from build123d import *

# Parameters (mm, degrees)
SKETCH_1_R           = 305
EXTRUDE_1_DEPTH      = 41.2
SKETCH_4_W           = 140
SKETCH_4_H           = 140
EXTRUDE_2_DEPTH      = 10
SHELL_1_T            = -5
CUT_EXTRUDE_3_DEPTH  = 434.298326791
SKETCH_5_R           = 8
SKETCH_5_R_2         = 4
CUT_EXTRUDE_6_DEPTH  = 435.363258115
SKETCH_11_W          = 130
SKETCH_11_H          = 10
EXTRUDE_3_DEPTH      = 200
CUT_EXTRUDE_8_DEPTH  = 664.812051713
SKETCH_14_R          = 20
EXTRUDE_4_DEPTH      = 10
SKETCH_16_R          = 10
CUT_EXTRUDE_10_DEPTH = 626.006271969
SKETCH_19_W          = 5
SKETCH_19_H          = 36
EXTRUDE_5_DEPTH      = 26
CUT_EXTRUDE_11_DEPTH = 536.715493522
SKETCH_21_W          = 19
SKETCH_21_H          = 5
SKETCH_21_W_2        = 5
SKETCH_21_H_2        = 51.5


with BuildPart() as part:
    # 草图1 → 凸台-拉伸1 (new body)
    with BuildSketch(Plane(origin=(0, 0, 0), x_dir=(1, 0, 0), z_dir=(0, 1, 0))):
        with Locations(Location((0, 0, 0), (0, 0, 90))):
            Circle(SKETCH_1_R)
    extrude(amount=EXTRUDE_1_DEPTH)

    # 草图4 → 凸台-拉伸2 (add)
    with BuildSketch(Plane(origin=(0, 41.2, 0), x_dir=(1, 0, 0), z_dir=(0, 1, 0))):
        with Locations((183, 0)):
            Rectangle(SKETCH_4_W, SKETCH_4_H)
    extrude(amount=EXTRUDE_2_DEPTH)

    # 抽壳1
    shell_1_openings = [part.faces().sort_by_distance(p)[0] for p in [
        (0, 0, 0),
    ]]
    offset(amount=SHELL_1_T, openings=shell_1_openings, kind=Kind.INTERSECTION)

    # 草图2 → 切除-拉伸3 (cut, through all)
    with BuildSketch(Plane(origin=(0, 41.2, 0), x_dir=(1, 0, 0), z_dir=(0, 1, 0))):
        with BuildLine():
            Line((-182, -24), (-118, -24))
            ThreePointArc((-118, -24), (-100, -42), (-118, -60))
            Line((-118, -60), (-182, -60))
            ThreePointArc((-182, -60), (-200, -42), (-182, -24))
        make_face()
    extrude(amount=-CUT_EXTRUDE_3_DEPTH, mode=Mode.SUBTRACT)

    # 草图5 → 切除-拉伸6 (cut, through all)
    with BuildSketch(Plane(origin=(0, 51.2, 0), x_dir=(1, 0, 0), z_dir=(0, 1, 0))):
        with Locations(Location((183, 0, 0), (0, 0, 270))):
            Circle(SKETCH_5_R)
        with Locations(Location((129, 54, 0), (0, 0, 270))):
            Circle(SKETCH_5_R_2)
        with Locations(Location((237, 54, 0), (0, 0, 270))):
            Circle(SKETCH_5_R_2)
        with Locations(Location((237, -54, 0), (0, 0, 270))):
            Circle(SKETCH_5_R_2)
        with Locations(Location((129, -54, 0), (0, 0, 270))):
            Circle(SKETCH_5_R_2)
    extrude(amount=-CUT_EXTRUDE_6_DEPTH, mode=Mode.SUBTRACT)

    # 草图11 → 凸台-拉伸3 (add)
    with BuildSketch(Plane(origin=(0, 41.2, 0), x_dir=(1, 0, 0), z_dir=(0, 1, 0))):
        with Locations((104, 238)):
            Rectangle(SKETCH_11_W, SKETCH_11_H)
    extrude(amount=EXTRUDE_3_DEPTH)

    # 草图13 → 切除-拉伸8 (cut, through all)
    with BuildSketch(Plane.XY.offset(-233)):
        with BuildLine():
            Line((39, 41.2), (39, 241.2))
            Line((39, 241.2), (169, 241.2))
            Line((169, 241.2), (169, 41.2))
            Line((169, 41.2), (131, 41.2))
            ThreePointArc((131, 41.2), (138.32356193, 70.621084147), (140.99801314, 100.821780537))
            ThreePointArc((140.99801314, 100.821780537), (115.26317996, 135.706044936), (74.646786984, 120.556716136))
            ThreePointArc((74.646786984, 120.556716136), (53.931588882, 82.177347592), (39, 41.2))
        make_face()
    extrude(amount=-CUT_EXTRUDE_8_DEPTH, mode=Mode.SUBTRACT)

    # 草图14 → 凸台-拉伸4 (add)
    with BuildSketch(Plane.XY.offset(-233)):
        with Locations(Location((105, 101.2, 0), (0, 0, 180))):
            Circle(SKETCH_14_R)
    extrude(amount=EXTRUDE_4_DEPTH)

    # 草图16 → 切除-拉伸10 (cut, through all)
    with BuildSketch(Plane.XY.offset(-223)):
        with Locations((105, 101.2)):
            Circle(SKETCH_16_R)
    extrude(amount=-CUT_EXTRUDE_10_DEPTH, mode=Mode.SUBTRACT)

    # 草图19 → 凸台-拉伸5 (add)
    with BuildSketch(Plane.XY.offset(-233)):
        with Locations((75, 59.2)):
            Rectangle(SKETCH_19_W, SKETCH_19_H)
        with Locations((111, 59.2)):
            Rectangle(SKETCH_19_W, SKETCH_19_H)
    extrude(amount=EXTRUDE_5_DEPTH)

    # 草图20 → 切除-拉伸11 (cut, through all)
    with BuildSketch(Plane(origin=(113.5, 0, 0), x_dir=(0, 0, -1), z_dir=(1, 0, 0))):
        Polygon((233, 77.2), (207, 41.2), (207, 77.2), align=None)
    extrude(amount=-CUT_EXTRUDE_11_DEPTH, mode=Mode.SUBTRACT)

    # 草图21 → 旋转2 (revolve)
    with BuildSketch(Plane.XY, mode=Mode.PRIVATE) as revolve_2_sk:
        with Locations((-65.5, 33.7)):
            Rectangle(SKETCH_21_W, SKETCH_21_H)
        with Locations((-82.5, 10.45)):
            Rectangle(SKETCH_21_W_2, SKETCH_21_H_2)
    revolve(revolve_2_sk.sketch.rotate(Axis((0, 0, 0), (0, -1, 0)), 270), axis=Axis((0, 0, 0), (0, -1, 0)))


solid = part.part
Read the model definition and answer for the solid it produces. Units are mm, in the model's axes. A direction names the side the tool comes from. Coordinates: 2 decimals unless noted, no trailing zeros. Loops run counter-clockwise (first coordinate to the right, second up) from the corner with the lowest first, then second, coordinate; pieces in that order, holes last. Notation, with made-up numbers: (29.5, 54.5) -> (68.5, 54.5) arc R19 cw to (68.5, 89.5) -> close; hole circle Ø2 at (40.5, -26). An arc over 180 degrees is marked (long way). Answer in a Markdown table with one row per item.
Item 1: A cutting plane is placed at D-D on z = 224.5. Determine the outline of the cut face in (x, y), plus the area to 3 significant figures.
Returned:
| item | result |
|---|---|
| outline | (-206.46, 0) -> (-199, 0) -> (-199, 36.2) -> (199, 36.2) -> (199, 0) -> (206.46, 0) -> (206.46, 41.2) -> (-206.46, 41.2) -> close |
| area | 2,600 mm^2 |
Item 2: Each of these flat-tipped pins is pushed along its axis until it touches: P1, Ø4, axis at x = -142, y = 38.5, coming from the +Z side; P2, Ø8, axis at x = -33.5, z = 160, coming from the -Y side; P3, Ø2, axis at x = 141, y = 18.5, coming from the -Z side; P4, Ø5, axis at x = 129, z = 54, coming from the +Y side. Where does it stop, or does it pass through?
Returned:
| item | result |
|---|---|
| P1 | stops at z = 270.97 |
| P2 | stops at y = 36.2 |
| P3 | stops at z = -270.97 |
| P4 | passes through |
Item 3: For faces 1 (the flat face through (-1, 36.2, 1)), 2 (the flat face through (72.5, 55, -223)), 3 (the flat face through (101, 78, -243)), 4 (the cylindrical face through (-100, 39, 42)), determine the directions among +Z, -Z, +X, -X, +Y, -Y from which every point of the face is accessible in a straight line to the end or side of a thin tool.
Returned:
| item | result |
|---|---|
| face 1 | -Y |
| face 2 | +Z, -X, +Y |
| face 3 | -Z, +X, -X, +Y |
| face 4 | +Y, -Y |
Item 4: Straight lines are drawn through the part: line 1 along X through (y, z) = (48, -54); line 2 along X through (y, z) = (34.45, 0); line 3 along Y through (x, z) = (105, -224). For each, find the intervals that lie inside material, in ascending order. Write a range as [from, to].
Returned:
| item | result |
|---|---|
| line 1 | x = [113, 125], [133, 233], [241, 253] |
| line 2 | x = [-305, -300], [-85, -80], [-75, -56], [56, 75], [80, 85], [300, 305] |
| line 3 | y = [36.2, 41.2], [81.2, 91.2], [111.2, 121.2] |
Item 5: A cutting plane is placed at A-A on y = 9. Determine the outline of the cut face in (x, z).
Returned:
| item | result |
|---|---|
| outline | circle Ø610 at (0, 0); circle Ø170 at (0, 0); hole circle Ø600 at (0, 0); hole circle Ø160 at (0, 0) |
Item 6: A cutting plane is placed at C-C on x = 152.5. Determine the outline of the cut face in (y, z), plus the area to 3 significant figures.
Returned:
| item | result |
|---|---|
| outline | (0, -264.14) -> (41.2, -264.14) -> (41.2, -70) -> (51.2, -70) -> (51.2, 70) -> (41.2, 70) -> (41.2, 264.14) -> (0, 264.14) -> (0, 258.35) -> (36.2, 258.35) -> (36.2, 65) -> (46.2, 65) -> (46.2, -65) -> (36.2, -65) -> (36.2, -258.35) -> (0, -258.35) -> close |
| area | 3,160 mm^2 |
Item 7: For a pull along Z with two mould halves and no side action, classify faces 5 (the cylindrical face through (182.545, 17.847, 238.07)), 6 (the flat face through (5, 31.2, -56)), 7 (the flat face through (198, 51.2, -1)), 8 (the flat face through (114, 96, -223)) as released by +Z, released by -Z, zero draft, split by the parting line, or undercut.
Returned:
| item | result |
|---|---|
| face 5 | undercut |
| face 6 | undercut |
| face 7 | zero draft |
| face 8 | released by +Z |
Item 8: A cutting plane is placed at B-B on z = -101. Determine the outline of the cut face in (x, y).
Returned:
| item | result |
|---|---|
| outline | (-287.79, 0) -> (-282.49, 0) -> (-282.49, 36.2) -> (282.49, 36.2) -> (282.49, 0) -> (287.79, 0) -> (287.79, 41.2) -> (-287.79, 41.2) -> close |
